```python
from build123d import *

# Parameters (mm, degrees)
SKETCH1_W             = 35
SKETCH1_H             = 35
BOSS_EXTRUDE1_DEPTH   = 3
SKETCH3_W             = 25
SKETCH3_H             = 25
CUT_EXTRUDE1_DEPTH    = 4
SKETCH4_W             = 5
SKETCH4_H             = 4.1
SKETCH4_W_2           = 4.1
SKETCH4_H_2           = 5
CUT_EXTRUDE2_DEPTH    = 0.4
CHAMFER1_SIZE         = 0.75
CHAMFER1_SIZE2        = 2.060608065
CHAMFER1_PART_2_SIZE  = 0.75
CHAMFER1_PART_2_SIZE2 = 2.060608065
CHAMFER1_PART_3_SIZE  = 0.75
CHAMFER1_PART_3_SIZE2 = 2.060608065
CHAMFER1_PART_4_SIZE  = 0.75
CHAMFER1_PART_4_SIZE2 = 2.060608065
SKETCH6_R             = 1.1
CUT_EXTRUDE5_DEPTH    = 4
CUT_EXTRUDE6_DEPTH    = 1


with BuildPart() as part:
    # Sketch1 → Boss-Extrude1 (new body)
    with BuildSketch(Plane(origin=(0, 0, 0), x_dir=(1, 0, 0), z_dir=(0, 1, 0))):
        Rectangle(SKETCH1_W, SKETCH1_H)
    extrude(amount=BOSS_EXTRUDE1_DEPTH)

    # Sketch3 → Cut-Extrude1 (cut, through all)
    with BuildSketch(Plane(origin=(0, 3, 0), x_dir=(1, 0, 0), z_dir=(0, 1, 0))):
        Rectangle(SKETCH3_W, SKETCH3_H)
    extrude(amount=-CUT_EXTRUDE1_DEPTH, mode=Mode.SUBTRACT)

    # Sketch4 → Cut-Extrude2 (cut)
    with BuildSketch(Plane(origin=(0, 3, 0), x_dir=(1, 0, 0), z_dir=(0, 1, 0))):
        with Locations((-15, 3)):
            Rectangle(SKETCH4_W, SKETCH4_H)
        with Locations((-3, 15)):
            Rectangle(SKETCH4_W_2, SKETCH4_H_2)
        with Locations((3, 15)):
            Rectangle(SKETCH4_W_2, SKETCH4_H_2)
        with Locations((15, 3)):
            Rectangle(SKETCH4_W, SKETCH4_H)
        with Locations((15, -3)):
            Rectangle(SKETCH4_W, SKETCH4_H)
        with Locations((3, -15)):
            Rectangle(SKETCH4_W_2, SKETCH4_H_2)
        with Locations((-3, -15)):
            Rectangle(SKETCH4_W_2, SKETCH4_H_2)
        with Locations((-15, -3)):
            Rectangle(SKETCH4_W, SKETCH4_H)
    extrude(amount=-CUT_EXTRUDE2_DEPTH, mode=Mode.SUBTRACT)

    # Chamfer1
    chamfer1_edges = [part.edges().sort_by_distance(p)[0] for p in [
        (3, 2.6, 17.5),
        (-3, 2.6, 17.5),
    ]]
    chamfer1_side = [part.faces().sort_by_distance(p)[0] for p in [
        (0, 1.458081007, 17.5),
    ]]
    chamfer(chamfer1_edges, length=CHAMFER1_SIZE, length2=CHAMFER1_SIZE2, reference=chamfer1_side[0])

    # Chamfer1 part 2
    chamfer1_part_2_edges = [part.edges().sort_by_distance(p)[0] for p in [
        (-17.5, 2.6, 3),
        (-17.5, 2.6, -3),
    ]]
    chamfer1_part_2_side = [part.faces().sort_by_distance(p)[0] for p in [
        (-17.5, 1.458081007, 0),
    ]]
    chamfer(chamfer1_part_2_edges, length=CHAMFER1_PART_2_SIZE, length2=CHAMFER1_PART_2_SIZE2, reference=chamfer1_part_2_side[0])

    # Chamfer1 part 3
    chamfer1_part_3_edges = [part.edges().sort_by_distance(p)[0] for p in [
        (-3, 2.6, -17.5),
        (3, 2.6, -17.5),
    ]]
    chamfer1_part_3_side = [part.faces().sort_by_distance(p)[0] for p in [
        (0, 1.458081007, -17.5),
    ]]
    chamfer(chamfer1_part_3_edges, length=CHAMFER1_PART_3_SIZE, length2=CHAMFER1_PART_3_SIZE2, reference=chamfer1_part_3_side[0])

    # Chamfer1 part 4
    chamfer1_part_4_edges = [part.edges().sort_by_distance(p)[0] for p in [
        (17.5, 2.6, -3),
        (17.5, 2.6, 3),
    ]]
    chamfer1_part_4_side = [part.faces().sort_by_distance(p)[0] for p in [
        (17.5, 1.458081007, 0),
    ]]
    chamfer(chamfer1_part_4_edges, length=CHAMFER1_PART_4_SIZE, length2=CHAMFER1_PART_4_SIZE2, reference=chamfer1_part_4_side[0])

    # Sketch6 → Cut-Extrude5 (cut, through all)
    with BuildSketch(Plane(origin=(0, 3, 0), x_dir=(1, 0, 0), z_dir=(0, 1, 0))):
        with Locations((14.5, 14.5)):
            Circle(SKETCH6_R)
        with Locations((-14.5, 14.5)):
            Circle(SKETCH6_R)
        with Locations((-14.5, -14.5)):
            Circle(SKETCH6_R)
        with Locations((14.5, -14.5)):
            Circle(SKETCH6_R)
    extrude(amount=-CUT_EXTRUDE5_DEPTH, mode=Mode.SUBTRACT)

    # Sketch7 → Cut-Extrude6 (cut)
    with BuildSketch(Plane.XZ):
        Polygon((-12.867006838, 12.867006838), (-12.269289857, 15.097716981), (-13.902283019, 16.730710143), (-16.132993162, 16.132993162), (-16.730710143, 13.902283019), (-15.097716981, 12.269289857), align=None)
        Polygon((12.867006838, 12.867006838), (15.097716981, 12.269289857), (16.730710143, 13.902283019), (16.132993162, 16.132993162), (13.902283019, 16.730710143), (12.269289857, 15.097716981), align=None)
        Polygon((12.867006838, -12.867006838), (12.269289857, -15.097716981), (13.902283019, -16.730710143), (16.132993162, -16.132993162), (16.730710143, -13.902283019), (15.097716981, -12.269289857), align=None)
        Polygon((-12.867006838, -12.867006838), (-15.097716981, -12.269289857), (-16.730710143, -13.902283019), (-16.132993162, -16.132993162), (-13.902283019, -16.730710143), (-12.269289857, -15.097716981), align=None)
    extrude(amount=-CUT_EXTRUDE6_DEPTH, mode=Mode.SUBTRACT)


solid = part.part
```
Check sheet for the modelled part. Datum: model origin and axes. Units: mm. A direction names the side the tool comes from. Give positions to 0.01 mm unless a question says otherwise; leave off trailing zeros. Order: outer loops, then holes, each group sorted by start corner. A loop starts at its lowest first (then second) coordinate and runs counter-clockwise, first axis right, second up. Notation, with made-up numbers: M 28,-7 L 87,-7 A14 ccw 87,1 Z; hole C -21.5,53 d4. An arc over 180 degrees is marked long. Answer in a Markdown table with one row per item. Add a question column.
Q1. Sectioned sample at B-B, the plane x = 3.5. Record the boundary of the cut face in (y, z).
Q2. Thickness scan on L1, parallel to Z at x = -14.5, y = 2.1; L2, parallel to X at y = 2.65, z = 14.5. Record the ranges inside material, lowest first.
Q3. Sectioned sample at D-D, the plane x = -14.5. Record the boundary of the cut face in (y, z).
Q4. Gauge pin test, flat end, axial feed: pin 1 Ø1.5 at (x, z) = (-14.5, -2) entering from +Y. Record the tip position at first contact, or that the pin passes through.
Q5. Access from +Z, -Z, +X, -X, +Y, -Y to the whole of each face (thin tool, end or side, straight path). Record for faces 1 (the flat face through (0.95, 2.8, 15.6)), 2 (the flat face through (-16.46, 2.23, 3.03)), 3 (the flat face through (15.93, 0.49, -13.1)), 4 (the flat face through (0, 2, -12.5)).
Q6. Release check for a two-part mould opening along Z. For faces 5 (the flat face through (0, 3, 15)), 6 (the flat face through (-16.43, 0.49, 15.03)), 7 (the flat face through (-3.03, 2.23, -16.46)) record: released by +Z, released by -Z, zero draft, split by the parting line, or undercut.
Q7. Sectioned sample at C-C, the plane z = 14.5. Record the boundary of the cut face in (x, y).
Q8. Sectioned sample at A-A, the plane z = 10.5. Record the boundary of the cut face in (x, y).
Verdict:
| question | item | result |
|---|---|---|
| 1 | outline | M 0,-17.5 L 1.85,-17.5 L 2.6,-15.44 L 2.6,-12.5 L 0,-12.5 Z; M 0,12.5 L 2.6,12.5 L 2.6,15.44 L 1.85,17.5 L 0,17.5 Z |
| 2 | L1 | -17.5 to -15.6, -13.4 to 13.4, 15.6 to 17.5 |
| 2 | L2 | -17.5 to -15.6, -13.4 to -5.05, -0.95 to 0.95, 5.05 to 13.4, 15.6 to 17.5 |
| 3 | outline | M 0,-17.5 L 3,-17.5 L 3,-15.6 L 1,-15.6 L 1,-16.57 L 0,-16.57 Z; M 0,-12.43 L 1,-12.43 L 1,-13.4 L 3,-13.4 L 3,-5.05 L 2.6,-5.05 L 2.6,-0.95 L 3,-0.95 L 3,0.95 L 2.6,0.95 L 2.6,5.05 L 3,5.05 L 3,13.4 L 1,13.4 L 1,12.43 L 0,12.43 Z; M 0,16.57 L 1,16.57 L 1,15.6 L 3,15.6 L 3,17.5 L 0,17.5 Z |
| 4 | pin 1 | y = 2.6 |
| 5 | face 1 | +Z, +Y |
| 5 | face 2 | -X, +Y |
| 5 | face 3 | -Y |
| 5 | face 4 | +Y, -Y |
| 6 | face 5 | zero draft |
| 6 | face 6 | undercut |
| 6 | face 7 | released by -Z |
| 7 | outline | M -17.5,0 L -16.57,0 L -16.57,1 L -15.6,1 L -15.6,3 L -17.5,3 Z; M -13.4,1 L -12.43,1 L -12.43,0 L 12.43,0 L 12.43,1 L 13.4,1 L 13.4,3 L 5.05,3 L 5.05,2.6 L 0.95,2.6 L 0.95,3 L -0.95,3 L -0.95,2.6 L -5.05,2.6 L -5.05,3 L -13.4,3 Z; M 15.6,1 L 16.57,1 L 16.57,0 L 17.5,0 L 17.5,3 L 15.6,3 Z |
| 8 | outline | M -17.5,0 L -12.5,0 L -12.5,3 L -17.5,3 Z; M 12.5,0 L 17.5,0 L 17.5,3 L 12.5,3 Z |
